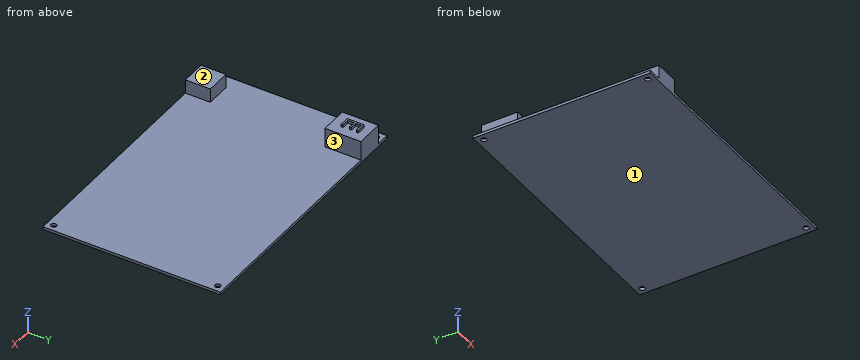
from build123d import *

# Parameters (mm, degrees)
F0_W     = 152.4
F0_H     = 101.6
F0_R     = 1.5875
F1_DEPTH = 1.5875
F2_W     = 15.875
F2_H     = 20.6375
F3_DEPTH = 12.7
F4_W     = 14.2875
F4_H     = 14.288262
F5_DEPTH = 7.9375
F6_W     = 15.875
F6_H     = 20.6375
F7_DEPTH = 1.5875


with BuildPart() as f1:
    # F0 (on Top) → F1 (new body)
    with BuildSketch(Plane.XY):
        with Locations((76.2, 50.8)):
            Rectangle(F0_W, F0_H)
        with Locations((3.8099971771, 3.8099971771)):
            Circle(F0_R, mode=Mode.SUBTRACT)
        with Locations((148.5900028229, 3.8099971771)):
            Circle(F0_R, mode=Mode.SUBTRACT)
        with Locations((3.8099971771, 97.7900028229)):
            Circle(F0_R, mode=Mode.SUBTRACT)
        with Locations((148.5900028229, 97.7900028229)):
            Circle(F0_R, mode=Mode.SUBTRACT)
    extrude(amount=F1_DEPTH)

    # F2 (on face) → F3 (join)
    with BuildSketch(Plane.XY.offset(1.5875)):
        with Locations((15.875, 91.28125)):
            Rectangle(F2_W, F2_H)
    extrude(amount=F3_DEPTH)

    # F4 (on face) → F5 (join)
    with BuildSketch(Plane.XY.offset(1.5875)):
        with Locations((15.08125, 7.144131)):
            Rectangle(F4_W, F4_H)
    extrude(amount=F5_DEPTH)

    # F6 (on face) → F7 (cut)
    with BuildSketch(Plane.XY.offset(14.2875)):
        with Locations((15.875, 91.28125)):
            Rectangle(F6_W, F6_H)
        Polygon((18.5745110599, 88.026480759), (18.5745110599, 87.0124623179), (13.1372374405, 87.0124623179), (13.1372374405, 96.7662523326), (18.5745110599, 96.7662523326), (18.5745110599, 95.7586382186), (14.2708033187, 95.7586382186), (14.2708033187, 92.6162484393), (18.3140684288, 92.6162484393), (18.3140684288, 91.6150386523), (14.2708033187, 91.6150386523), (14.2708033187, 88.026480759), align=None, mode=Mode.SUBTRACT)
    extrude(amount=-F7_DEPTH, mode=Mode.SUBTRACT)


solid = f1.part
Geometry: final body of the model. Coordinates: model frame, mm. Face numbers are marked on the shaded views. A direction names the side the tool comes from. Round coordinates to 2 decimals unless told otherwise and drop trailing zeros. Loops run counter-clockwise (first coordinate to the right, second up) from the corner with the lowest first, then second, coordinate; pieces in that order, holes last. Notation, with made-up numbers: (42, 55) - (82, 55) arc R4 ccw to (82, 60) - close; hole circle Ø4 at (76, -6). An arc over 180 degrees is marked (long way). Write each question's results on one line, items separated by ' | '. Start each with the question number.
1) Cut plane D-D on x = 131. Return loops of the section in (y, z).
2) Cut plane C-C on y = 85. Return loops of the section in (x, z), then the cut area to 3 significant figures.
3) First-contact query: P1, Ø1.1, axis at y = 87.5, z = 13.5, coming from the +X side; P2, Ø1.5, axis at y = 76, z = 3.5, coming from the +X side; P3, Ø0.8, axis at y = 94.5, z = 13.5, coming from the +X side; P4, Ø0.8, axis at y = 92, z = 13.5, coming from the +X side. Flat tips, straight axial feed; report the tip coordinate or a pass-through.
4) Line query: probe 1 along Z at (x, y) = (119.5, 41); probe 2 along X at (y, z) = (12.5, 2.75) (1 decimal); probe 3 along Z at (x, y) = (8.5, 13) (3 decimals). Output: solid intervals per line, ascending. Write a range as [from, to].
5) Cut plane A-A on z = 6.5. Return loops of the section in (x, y) (1 decimal).
6) Cut plane B-B on x = 16. Return loops of the section in (y, z) (1 decimal).
7) Access query for the marked faces 1, 2 and 3. Directions: +Z, -Z, +X, -X, +Y, -Y. A direction counts if a zero-diameter tool reaches every point of the face in a straight line with its end or side. Return the directions, or none.
Verdict:
1) outline: (0, 0) - (101.6, 0) - (101.6, 1.59) - (0, 1.59) - close
2) outline: (0, 0) - (152.4, 0) - (152.4, 1.59) - (23.81, 1.59) - (23.81, 12.7) - (7.94, 12.7) - (7.94, 1.59) - (0, 1.59) - close | area: 418 mm2
3) P1: stops at x = 18.57 | P2: passes through | P3: stops at x = 14.27 | P4: stops at x = 18.31
4) probe 1: z = [0, 1.59] | probe 2: x = [7.9, 22.2] | probe 3: z = [0, 9.525]
5) outline: (7.9, 0) - (22.2, 0) - (22.2, 14.3) - (7.9, 14.3) - close; (7.9, 81) - (23.8, 81) - (23.8, 101.6) - (7.9, 101.6) - close
6) outline: (0, 0) - (101.6, 0) - (101.6, 12.7) - (96.8, 12.7) - (96.8, 14.3) - (95.8, 14.3) - (95.8, 12.7) - (92.6, 12.7) - (92.6, 14.3) - (91.6, 14.3) - (91.6, 12.7) - (88, 12.7) - (88, 14.3) - (87, 14.3) - (87, 12.7) - (81, 12.7) - (81, 1.6) - (14.3, 1.6) - (14.3, 9.5) - (0, 9.5) - close
7) face 1: -Z, +X, -X, +Y, -Y | face 2: +Z, +X, -X, -Y | face 3: +Z, +X, +Y, -Y
